Here's how the part is built. I have some questions about the finished solid (model axes, mm). Face numbers are marked on the shaded views. A direction names the side the tool comes from. Coordinates: 2 decimals unless noted, no trailing zeros. Loops run counter-clockwise (first coordinate to the right, second up) from the corner with the lowest first, then second, coordinate; pieces in that order, holes last. Notation, with made-up numbers: M 42.5,11 L 82.5,11 A30 cw 82.5,48 Z; hole C 54,77.5 d4. An arc over 180 degrees is marked long. Use one line per item in the form item = value. Start each with the question number.
(1) Imagine slicing it at C-C, the plane z = -19. Please give me the cut outline in (x, y).
(2) Imagine slicing it at D-D, the plane z = 28. Please give me the cut outline in (x, y) (3 decimals), and give its area (3 significant figures).
(3) Imagine slicing it at A-A, the plane x = 0. Please give me the cut outline in (y, z), and give its area (3 significant figures).
(4) Imagine slicing it at B-B, the plane y = 6.5. Please give me the cut outline in (x, z), and give its area (3 significant figures).
(5) Please list where these lines run through material, in increasing order: L1, parallel to Z at x = 0, y = 8.5; L2, parallel to Y at x = 13.5, z = 7; L3, parallel to Z at x = 24.5, y = 43.5.
(6) On a 3-axis mill with a long thin cutter (end or side, diameter ignored), from which of +Z, -Z, +X, -X, +Y, -Y can I reach the whole of each face in a straight line? I mean the marked faces 1, 2, 3 and 4. Say none if no direction works.
(7) Thinking about a two-plate mould opening in X: for the marked faces 5, 6 and 7, which applies, +X half, -X half, draft (parallel to the pull), parting line (faces both ways), or undercut?
(8) Will these pins go through, and if not, where does the flat tip stop? P1, Ø2, axis at x = -25, y = 11.5, coming from the +Z side; P2, Ø12, axis at x = -7.5, y = 49, coming from the +Z side; P3, Ø24, axis at y = 51.5, z = -20.5, coming from the +X side; P4, Ø11, axis at y = 22.5, z = 46, coming from the +X side.
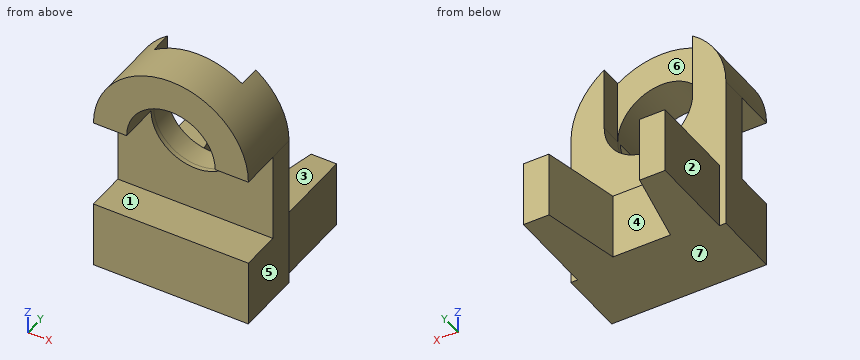
```python
from build123d import *

# Parameters (mm, degrees)
SKETCH1_R           = 20
SKETCH1_W           = 70
SKETCH1_H           = 30
BOSS_EXTRUDE1_DEPTH = 30
SKETCH2_W           = 40
SKETCH2_H           = 18
CUT_EXTRUDE1_DEPTH  = 70
CUT_EXTRUDE2_START  = -10
CUT_EXTRUDE2_DEPTH  = 10
SKETCH4_W           = 64
SKETCH4_H           = 30
BOSS_EXTRUDE2_DEPTH = 40
CUT_EXTRUDE3_DEPTH  = 109.397416943


with BuildPart() as part:
    # Sketch1 → Boss-Extrude1 (new body)
    # profile 1 of 2: a face of its own
    with BuildSketch(Plane(origin=(0, 0, 0), x_dir=(1, 0, 0), z_dir=(0, 1, 0))):
        with BuildLine():
            Line((-35, 5), (-35, -35))
            ThreePointArc((-35, -35), (0, -70), (35, -35))
            Line((35, -35), (35, 5))
            Line((35, 5), (-35, 5))
        make_face()
        with Locations(Location((0, -35, 0), (0, 0, 270))):
            Circle(SKETCH1_R, mode=Mode.SUBTRACT)
    # profile 2 of 2: a face of its own
    with BuildSketch(Plane(origin=(0, 0, 0), x_dir=(1, 0, 0), z_dir=(0, 1, 0))):
        with Locations((0, 20)):
            Rectangle(SKETCH1_W, SKETCH1_H)
    extrude(amount=BOSS_EXTRUDE1_DEPTH)

    # Sketch2 → Cut-Extrude1 (cut)
    with BuildSketch(Plane(origin=(35, 0, 0), x_dir=(0, 0, -1), z_dir=(1, 0, 0))):
        with Locations((-15, 9)):
            Rectangle(SKETCH2_W, SKETCH2_H)
    extrude(amount=-CUT_EXTRUDE1_DEPTH, mode=Mode.SUBTRACT)

    # Sketch3 → Cut-Extrude2 (cut)
    with BuildSketch(Plane(origin=(0, 30, 0), x_dir=(1, 0, 0), z_dir=(0, 1, 0)).offset(CUT_EXTRUDE2_START)):
        with BuildLine():
            Line((20, -35), (20, -91.691085181))
            Line((20, -91.691085181), (-20, -91.691085181))
            Line((-20, -91.691085181), (-20, -35))
            ThreePointArc((-20, -35), (0, -15), (20, -35))
        make_face()
    extrude(amount=CUT_EXTRUDE2_DEPTH, mode=Mode.SUBTRACT)

    # Sketch4 → Boss-Extrude2 (add)
    with BuildSketch(Plane(origin=(0, 30, 0), x_dir=(1, 0, 0), z_dir=(0, 1, 0))):
        with Locations((0, 20)):
            Rectangle(SKETCH4_W, SKETCH4_H)
    extrude(amount=BOSS_EXTRUDE2_DEPTH)

    # Sketch5 → Cut-Extrude3 (cut, through all)
    with BuildSketch(Plane.XY.offset(-5)):
        Polygon((-20.5, 70), (20.5, 70), (13, 35), (-13, 35), align=None)
    extrude(amount=-CUT_EXTRUDE3_DEPTH, mode=Mode.SUBTRACT)


solid = part.part
```
Answer:
q1.outline = M -35,0 L 35,0 L 35,30 L 32,30 L 32,70 L 20.5,70 L 13,35 L -13,35 L -20.5,70 L -32,70 L -32,30 L -35,30 Z
q2.outline = M -35,18 L -18.735,18 L -18.735,30 L -35,30 Z; M 18.735,18 L 35,18 L 35,30 L 18.735,30 Z
q2.area = 390 mm²
q3.outline = M 0,-35 L 35,-35 L 35,-5 L 30,-5 L 30,15 L 18,15 L 18,-5 L 0,-5 Z; M 0,55 L 20,55 L 20,70 L 0,70 Z
q3.area = 1,590 mm²
q4.outline = M -35,-35 L 35,-35 L 35,-5 L -35,-5 Z; M -35,35 L -20,35 A20 cw 20,35 L 35,35 A35 ccw Z
q4.area = 3,400 mm²
q5.L1 = -35 to -5, 55 to 70
q5.L2 = 18 to 30
q5.L3 = -35 to -5
q6.face_1 = +X, -X, -Y
q6.face_2 = +Z, -Z, -X, +Y
q6.face_3 = +Z, +X, -X, +Y
q6.face_4 = +Z, -Z, +Y
q7.face_5 = +X half
q7.face_6 = undercut
q7.face_7 = draft
q8.P1 = 60.48
q8.P2 = through
q8.P3 = 32
q8.P4 = 34.57
